Read the model definition and answer for the solid it produces. Units are mm, in the model's axes. Round coordinates to 2 decimals unless told otherwise and drop trailing zeros. Order: outer loops, then holes, each group sorted by start corner. A loop starts at its lowest first (then second) coordinate and runs counter-clockwise, first axis right, second up. Notation, with made-up numbers: (81.5, 14.25) -> (131.5, 14.25) arc R20 cw to (131.5, 29.25) -> close; hole circle Ø1 at (-2.75, -1). An arc over 180 degrees is marked (long way). Answer as a JSON object with one key per item and string values. Group by question number.
Item 1: Section C-C, the plane y = 1 is taken. Write down the section's boundary in (x, z), plus the area to 3 significant figures.
Item 2: Section A-A, the plane x = -3.75 is taken. Write down the section's boundary in (y, z).
Item 3: Section B-B, the plane z = 9 is taken. Write down the section's boundary in (x, y), plus the area to 3 significant figures.
Item 4: Consider probe 1 along Z at (x, y) = (-4, 3.5); probe 2 along Z at (x, y) = (0.75, -3.25); probe 3 along X at (y, z) = (4.75, 9). Determine where each line is inside the solid, lowest interval first. Write a range as from..to.
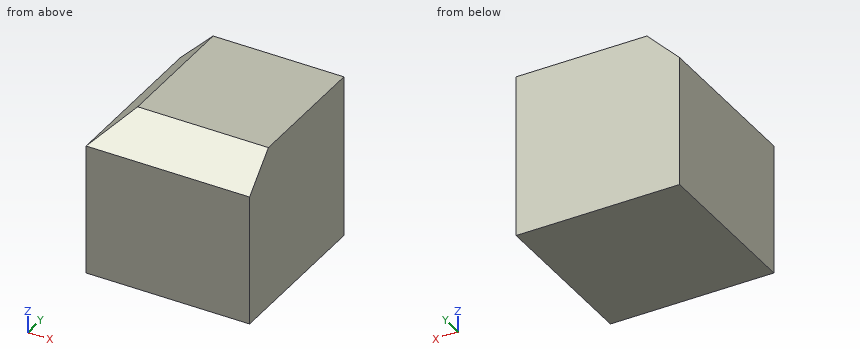
from build123d import *

# Parameters (mm, degrees)
SKETCH1_W           = 10
SKETCH1_H           = 10
BOSS_EXTRUDE1_DEPTH = 10
CHAMFER1_SIZE       = 2


with BuildPart() as part:
    # Sketch1 → Boss-Extrude1 (new body)
    with BuildSketch(Plane.XY):
        Rectangle(SKETCH1_W, SKETCH1_H)
    extrude(amount=BOSS_EXTRUDE1_DEPTH)

    # Chamfer1
    chamfer1_edges = [part.edges().sort_by_distance(p)[0] for p in [
        (0, -5, 10),
        (-5, 0, 10),
    ]]
    chamfer(chamfer1_edges, length=CHAMFER1_SIZE)


solid = part.part
Values found:
{
 "1": {"outline": "(-5, 0) -> (5, 0) -> (5, 10) -> (-3, 10) -> (-5, 8) -> close", "area": "98.0 mm2"},
 "2": {"outline": "(-5, 0) -> (5, 0) -> (5, 9.25) -> (-3.75, 9.25) -> (-5, 8) -> close"},
 "3": {"outline": "(-4, -4) -> (5, -4) -> (5, 5) -> (-4, 5) -> close", "area": "81.0 mm2"},
 "4": {"probe 1": "0..9", "probe 2": "0..9.75", "probe 3": "-4..5"}
}
